Autodesk Fusion 360 part; units mm, degrees
sketch "スケッチ1" plane through (0, 0, 0) normal (0, 0, 1) x (1, 0, 0)
  line L0 (0, 0) -> (20, 0)
  line L1 (20, 0) -> (20, 23)
  line L2 (20, 23) -> (0, 23)
  line L3 (0, 23) -> (0, 0)
  dimension "d1" = 20
  dimension "d2" = 23
extrude "押し出し1" add sketch "スケッチ1" along normal blind 2
sketch "スケッチ2" plane through (0, 0, 2) normal (0, 0, 1) x (-1, 0, 0)
  line L0 (0, -23) -> (0, 0)
  line L1 (0, 0) -> (-20, 0)
  line L2 (-20, 0) -> (-20, -23)
  line L3 (-20, -23) -> (0, -23)
  line L4 (0, -23) -> (-5, -23)
  line L5 (-5, -23) -> (-5, -18)
  line L6 (-5, -18) -> (0, -18)
  line L7 (0, -18) -> (0, -23)
  line L8 (-20, -23) -> (-15, -23)
  line L9 (-15, -23) -> (-15, -18)
  line L10 (-15, -18) -> (-20, -18)
  line L11 (-20, -18) -> (-20, -23)
  line L12 (0, 0) -> (-5, 0)
  line L13 (-5, 0) -> (-5, -5)
  line L14 (-5, -5) -> (0, -5)
  line L15 (0, -5) -> (0, 0)
  line L16 (-20, 0) -> (-15, 0)
  line L17 (-15, 0) -> (-15, -5)
  line L18 (-15, -5) -> (-20, -5)
  line L19 (-20, -5) -> (-20, 0)
  line L20 (-2, -21) -> (-18, -21)
  line L21 (-18, -21) -> (-18, -2)
  line L22 (-18, -2) -> (-2, -2)
  line L23 (-2, -2) -> (-2, -21)
  dimension "d5" = 5
  dimension "d6" = 5
  dimension "d7" = 5
  dimension "d8" = 5
  dimension "d9" = 5
  dimension "d10" = 5
  dimension "d11" = 5
  dimension "d12" = 5
extrude "押し出し2" add sketch "スケッチ2" along normal blind 2 contours L0 L3 L4 L5 L6 L7 L20 L23 | L0 L1 L12 L13 L14 L15 L22 L23 | L5 L6 L20 L23 | L5 L6 L9 L10 L13 L14 L17 L18 L20 L21 L22 L23 | L2 L3 L8 L9 L10 L11 L20 L21 | L13 L14 L22 L23 | L9 L10 L20 L21 | L1 L2 L16 L17 L18 L19 L21 L22 | L17 L18 L21 L22
sketch "スケッチ3" plane through (0, 0, 4) normal (0, 0, 1) x (-1, 0, 0)
  line L0 (-18, -18) -> (-20, -18)
  line L1 (-20, -18) -> (-20, -23)
  line L2 (-20, -23) -> (-15, -23)
  line L3 (-15, -23) -> (-15, -21)
  line L4 (-15, -21) -> (-5, -21)
  line L5 (-5, -21) -> (-5, -23)
  line L6 (-5, -23) -> (0, -23)
  line L7 (0, -23) -> (0, -18)
  line L8 (0, -18) -> (-2, -18)
  line L9 (-2, -18) -> (-2, -5)
  line L10 (-2, -5) -> (0, -5)
  line L11 (0, -5) -> (0, 0)
  line L12 (0, 0) -> (-5, 0)
  line L13 (-5, 0) -> (-5, -2)
  line L14 (-5, -2) -> (-15, -2)
  line L15 (-15, -2) -> (-15, 0)
  line L16 (-15, 0) -> (-20, 0)
  line L17 (-20, 0) -> (-20, -5)
  line L18 (-20, -5) -> (-18, -5)
  line L19 (-18, -5) -> (-18, -18)
  line L20 (-5, -18) -> (-15, -18)
  line L21 (-15, -18) -> (-15, -5)
  line L22 (-15, -5) -> (-5, -5)
  line L23 (-5, -5) -> (-5, -18)
extrude "押し出し3" add sketch "スケッチ3" along normal blind 3 contours L20 L21 L22 L23
sketch "スケッチ4" plane through (0, 0, 7) normal (0, 0, 1) x (-1, 0, 0)
  line L0 (-5, -5) -> (-15, -5)
  line L1 (-15, -5) -> (-15, -18)
  line L2 (-15, -18) -> (-5, -18)
  line L3 (-5, -18) -> (-5, -5)
  line L4 (-9.55, -13.5) -> (-11.05, -13.5)
  line L5 (-11.05, -13.5) -> (-11.05, -9.5)
  line L6 (-11.05, -9.5) -> (-9.55, -9.5)
  line L7 (-9.55, -9.5) -> (-9.55, -13.5)
  line L8 (-8.3, -12.25) -> (-12.3, -12.25)
  line L9 (-12.3, -12.25) -> (-12.3, -10.75)
  line L10 (-12.3, -10.75) -> (-8.3, -10.75)
  line L11 (-8.3, -10.75) -> (-8.3, -12.25)
  circle A0 centre (-10.3, -11.5) radius 2.75
  dimension "d17" = 13
  dimension "d18" = 1.5
  dimension "d19" = 4
  dimension "d20" = 4
  dimension "d21" = 1.5
  dimension "d22" = 5.5
extrude "押し出し4" add sketch "スケッチ4" along normal blind 3.5 contours A0
sketch "スケッチ5" plane through (0, 0, 0) normal (0, 0, -1) x (1, 0, 0)
  line L0 (0, 0) -> (0, -23)
  line L1 (0, -23) -> (20, -23)
  line L2 (20, -23) -> (20, 0)
  line L3 (20, 0) -> (0, 0)
  line L4 (16.5, -11.5) -> (13, -15)
  line L5 (13, -8) -> (16.5, -11.5)
  line L6 (13, -15) -> (5, -15)
  line L7 (5, -15) -> (5, -8)
  line L8 (5, -8) -> (13, -8)
  line L9 (7.3948, -12.9209) -> (10.9304, -9.3854)
  line L10 (11.6375, -10.0925) -> (8.102, -13.628)
  line L11 (8.102, -13.628) -> (7.3948, -12.9209)
  line L12 (10.9304, -9.3854) -> (11.6375, -10.0925)
  line L13 (7.3948, -10.0925) -> (8.102, -9.3854)
  line L14 (11.6375, -12.9209) -> (10.9304, -13.628)
  line L15 (10.9304, -13.628) -> (7.3948, -10.0925)
  line L16 (8.102, -9.3854) -> (11.6375, -12.9209)
extrude "押し出し5" cut sketch "スケッチ5" against normal blind 1 contours L4 L5 L6 L7 L8
The listing builds one solid part. Answer for the finished solid, in the listing's coordinates (mm). A direction names the side the tool comes from. Give positions to 0.01 mm unless a question says otherwise; leave off trailing zeros. Order: outer loops, then holes, each group sorted by start corner. A loop starts at its lowest first (then second) coordinate and runs counter-clockwise, first axis right, second up.
Item 1: The part is cut by section D-D, the plane z = 6.25. Give the vertices of the cut face in (x, y), and give its area (3 significant figures).
From the geometry:
outline: (5, 5) - (15, 5) - (15, 18) - (5, 18) - close
area: 130 mm2
Item 2: The part is cut by section B-B, the plane z = 8.5. Give the vertices of the cut face in (x, y).
From the geometry:
outline: circle Ø5.5 at (10.3, 11.5); hole (8.3, 10.75) - (9.55, 10.75) - (9.55, 9.5) - (11.05, 9.5) - (11.05, 10.75) - (12.3, 10.75) - (12.3, 12.25) - (11.05, 12.25) - (11.05, 13.5) - (9.55, 13.5) - (9.55, 12.25) - (8.3, 12.25) - close
Item 3: Which of the six approach directions +Z, -Z, +X, -X, +Y, -Y give full straight-line access (tool end or side, diameter ignored) to faces 5 (the face through (8.799, 10.083, 0.493)), 6 (the face through (10, 2, 3)), 7 (the face through (11.05, 13, 9))?
From the geometry:
face 5: -Z
face 6: +Z, -Y
face 7: +Z
Item 4: For a pull along X with two mould halves and no side action, classify faces 1 (the face through (15, 12, 5)), 2 (the face through (14.8, 13.2, 0.5)), 3 (the face through (19, 12, 2)), 4 (the face through (5, 1, 3)) as pulls with the +X half, pulls with the -X half, needs draft (parallel to the pull), parting line crosses it, or undercut.
From the geometry:
face 1: pulls with the +X half
face 2: undercut
face 3: needs draft
face 4: undercut
Item 5: The part is cut by section C-C, the plane x = 6.5. Give the vertices of the cut face in (y, z).
From the geometry:
outline: (0, 0) - (8, 0) - (8, 1) - (15, 1) - (15, 0) - (23, 0) - (23, 2) - (21, 2) - (21, 4) - (18, 4) - (18, 7) - (5, 7) - (5, 4) - (2, 4) - (2, 2) - (0, 2) - close
Item 6: Given pin 1 Ø0.6 at (x, y) = (18.5, 10.5) entering from +Z; pin 2 Ø0.9 at (y, z) = (8.5, 5) entering from -X; pin 3 Ø1.4 at (y, z) = (10, 8.5) entering from +X, each flat-ended and moving along its own axis, determine where each tip first touches the part or whether it passes through.
From the geometry:
pin 1: stops at z = 2
pin 2: stops at x = 5
pin 3: stops at x = 12.93
Item 7: Find the intervals of material crossed by probe 1 along Z at (x, y) = (4, 18.25); probe 2 along Z at (x, y) = (14.5, 7); probe 3 along X at (y, z) = (10, 3), in increasing order.
From the geometry:
probe 1: z = 0 to 4
probe 2: z = 0 to 7
probe 3: x = 2 to 18
Item 8: The part is cut by section A-A, the plane y = 5.5. Give the vertices of the cut face in (x, z).
From the geometry:
outline: (0, 0) - (20, 0) - (20, 2) - (18, 2) - (18, 4) - (15, 4) - (15, 7) - (5, 7) - (5, 4) - (2, 4) - (2, 2) - (0, 2) - close
